Could you check a few things on this model? Use its own coordinates, in mm. A direction names the side the tool comes from. Coordinates: 2 decimals unless noted, no trailing zeros. Order: outer loops, then holes, each group sorted by start corner. A loop starts at its lowest first (then second) coordinate and runs counter-clockwise, first axis right, second up. Notation, with made-up numbers: (-33.5, 33.5) -> (13.5, 33.5) arc R21 ccw to (13.5, 51.5) -> close; hole circle Ø3 at (9.25, 4). An arc over 180 degrees is marked (long way). Return JSON: item names as keys, results as strings. Group by question number.
Autodesk Inventor part; units mm, degrees
ref_plane "YZ Plane" through (0, 0, 0) normal (1, 0, 0) x (0, 1, 0)
ref_plane "XZ Plane" through (0, 0, 0) normal (0, 1, 0) x (-1, 0, 0)
ref_plane "XY Plane" through (0, 0, 0) normal (0, 0, 1) x (1, 0, 0)
sketch "Szkic1" plane through (0, 0, 0) normal (0, 0, 1) x (1, 0, 0)
  line L0 (0, 0) -> (21, 0)
  line L1 (21, 0) -> (21, 25)
  line L2 (21, 25) -> (0, 25)
  line L3 (0, 25) -> (0, 0)
  line L4 (21, 25) -> (26, 25)
  line L5 (26, 25) -> (26, 0)
  line L6 (26, 0) -> (21, 0)
  line L7 (21, 0) -> (21, 25)
  line L8 (0, 12.5) -> (26, 12.5) construction
  circle A0 centre (7.5, 17.5) radius 2.8
  circle A1 centre (7.5, 7.5) radius 2.8
  dimension "d0" = 21
  dimension "d1" = 25
  dimension "d2" = 5
  dimension "d4" = 7.5
  dimension "d5" = 5.6
  dimension "d13" = 10
extrude "Wyciągnięcie proste1" add sketch "Szkic1" along normal mid plane 52
extrude "Wyciągnięcie proste2" cut sketch "Szkic1" along normal mid plane 42 contours L3 L2 L1 L0
chamfer "Faza1" distance 5 angle 45 2 edges at (21, 12.5, 21) (21, 12.5, -21)
fillet "Zaokrąglenie1" radius 1.6 10 edges at (0, 12.5, 26) (0, 12.5, 21) (26, 12.5, 26) (26, 12.5, -26) (0, 12.5, -26) (0, 12.5, -21) (16, 12.5, 21) (21, 12.5, 16) (21, 12.5, -16) (16, 12.5, -21)
properties part number "finger_rig" material "PLA"
Q1. I want a section at C-C on x = 18.5. Please give me the cut outline in (y, z), and give its area (3 significant figures).
Q2. We'd pull the mould along Z, two halves only. Please class faces 3 (the cylindrical face through (20.875, 12.675, 15.958)), 4 (the flat face through (21.5, 0, -0.4)), 5 (the flat face through (13, 13, -26)): pulls with the +Z half, pulls with the -Z half, needs draft (parallel to the pull), parting line crosses it, or undercut.
Q3. I'm going to push flat-ended pins straight in: pin 1 Ø12.5 at (y, z) = (8, -4.5) entering from -X; pin 2 Ø7.5 at (x, y) = (7.5, 7.5) entering from -Z; pin 3 Ø5 at (x, y) = (7.5, 17.5) entering from +Z. Where does each tip first touch, or does it pass through?
Q4. I want a section at D-D on y = 11. Please give me the cut outline in (x, z), and give its area (3 significant figures).
Q5. I need wall thicknesses on line 1 along Y through (x, z) = (7.5, -23.45); line 2 along Z through (x, y) = (15.5, 23.25); line 3 along Z through (x, y) = (1, 7.5). Which ranges of each line are inside material? Lowest first, please. Write a range as from..to.
Q6. I want a section at A-A on x = 7.5. Please give me the cut outline in (y, z), and give its area (3 significant figures).
Q7. I want a section at B-B on y = 7.5. Please give me the cut outline in (x, z), and give its area (3 significant figures).
Q8. On a 3-axis mill with a long thin cutter (end or side, diameter ignored), from which of +Z, -Z, +X, -X, +Y, -Y can I reach the whole of each face in a straight line? I mean faces 1 (the cylindrical face through (15.958, 12.675, -20.875)), 2 (the flat face through (26, 13, 0)). Say none if no direction works.
Response values:
{
 "1": {"outline": "(0, -26) -> (25, -26) -> (25, -18.5) -> (0, -18.5) -> close; (0, 18.5) -> (25, 18.5) -> (25, 26) -> (0, 26) -> close", "area": "375 mm²"},
 "2": {"face 3": "undercut", "face 4": "needs draft", "face 5": "pulls with the -Z half"},
 "3": {"pin 1": "stops at x = 21", "pin 2": "stops at z = -26", "pin 3": "passes through"},
 "4": {"outline": "(0, -24.4) arc R1.6 ccw to (1.6, -26) -> (24.4, -26) arc R1.6 ccw to (26, -24.4) -> (26, 24.4) arc R1.6 ccw to (24.4, 26) -> (1.6, 26) arc R1.6 ccw to (0, 24.4) -> (0, 22.6) arc R1.6 ccw to (1.6, 21) -> (15.34, 21) arc R1.6 cw to (16.47, 20.53) -> (20.53, 16.47) arc R1.6 cw to (21, 15.34) -> (21, -15.34) arc R1.6 cw to (20.53, -16.47) -> (16.47, -20.53) arc R1.6 cw to (15.34, -21) -> (1.6, -21) arc R1.6 ccw to (0, -22.6) -> close", "area": "492 mm²"},
 "5": {"line 1": "y = 0..4.7, 10.3..14.7, 20.3..25", "line 2": "z = -26..-20.99, 20.99..26", "line 3": "z = -25.88..-21.12, 21.12..25.88"},
 "6": {"outline": "(0, -26) -> (4.7, -26) -> (4.7, -21) -> (0, -21) -> close; (0, 21) -> (4.7, 21) -> (4.7, 26) -> (0, 26) -> close; (10.3, -26) -> (14.7, -26) -> (14.7, -21) -> (10.3, -21) -> close; (10.3, 21) -> (14.7, 21) -> (14.7, 26) -> (10.3, 26) -> close; (20.3, -26) -> (25, -26) -> (25, -21) -> (20.3, -21) -> close; (20.3, 21) -> (25, 21) -> (25, 26) -> (20.3, 26) -> close", "area": "138 mm²"},
 "7": {"outline": "(0, -24.4) arc R1.6 ccw to (1.6, -26) -> (4.7, -26) -> (4.7, -21) -> (1.6, -21) arc R1.6 ccw to (0, -22.6) -> close; (0, 22.6) arc R1.6 ccw to (1.6, 21) -> (4.7, 21) -> (4.7, 26) -> (1.6, 26) arc R1.6 ccw to (0, 24.4) -> close; (10.3, -26) -> (24.4, -26) arc R1.6 ccw to (26, -24.4) -> (26, 24.4) arc R1.6 ccw to (24.4, 26) -> (10.3, 26) -> (10.3, 21) -> (15.34, 21) arc R1.6 cw to (16.47, 20.53) -> (20.53, 16.47) arc R1.6 cw to (21, 15.34) -> (21, -15.34) arc R1.6 cw to (20.53, -16.47) -> (16.47, -20.53) arc R1.6 cw to (15.34, -21) -> (10.3, -21) -> close", "area": "436 mm²"},
 "8": {"face 1": "-X, +Y, -Y", "face 2": "+Z, -Z, +X, +Y, -Y"}
}
